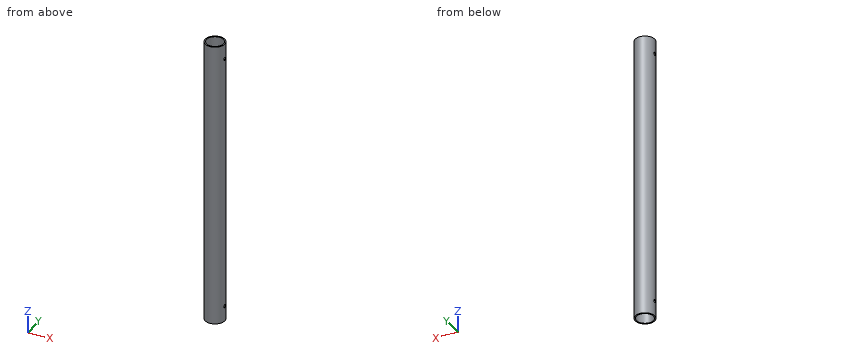
from build123d import *

# Parameters (mm, degrees)
F0_R          = 15.875
F0_R_2        = 13.875
F1_DEPTH      = 470
F2_R          = 2.5
F3_DEPTH      = 30
F3_DEPTH_BACK = 30
F4_R          = 2.5
F5_DEPTH      = 25
F5_DEPTH_BACK = 25


with BuildPart() as f1:
    # F0 (on Top) → F1 (new body)
    with BuildSketch(Plane.XY):
        Circle(F0_R)
        Circle(F0_R_2, mode=Mode.SUBTRACT)
    extrude(amount=F1_DEPTH)

    # F2 (on Right) → F3 (cut, two sides)
    with BuildSketch(Plane.YZ) as f3_sk:
        with Locations((0, 25)):
            Circle(F2_R)
    extrude(amount=F3_DEPTH, mode=Mode.SUBTRACT)
    extrude(f3_sk.sketch, amount=-F3_DEPTH_BACK, mode=Mode.SUBTRACT)

    # F4 (on Right) → F5 (cut, two sides)
    with BuildSketch(Plane.YZ) as f5_sk:
        with Locations((0, 445)):
            Circle(F4_R)
    extrude(amount=-F5_DEPTH, mode=Mode.SUBTRACT)
    extrude(f5_sk.sketch, amount=F5_DEPTH_BACK, mode=Mode.SUBTRACT)


solid = f1.part
Input: part model. Units: mm. Frame: model coordinates. Give positions to 0.01 mm unless a question says otherwise; leave off trailing zeros. Order: outer loops, then holes, each group sorted by start corner. A loop starts at its lowest first (then second) coordinate and runs counter-clockwise, first axis right, second up. Notation, with made-up numbers: M 38.5,7 L 53.5,7 A16 cw 53.5,15 Z; hole C -27.5,64 d7. An arc over 180 degrees is marked long. Answer as a JSON object with one key per item and string values.
1. Ray query, line 1 (Z direction, x = 15.3, y = 0); line 2 (X direction, y = -1.5, z = 406); line 3 (Y direction, x = 0, z = 104.5) (3 decimals). Return the intervals inside material, ascending. Write a range as [from, to].
Result sheet:
{"line 1": "[0, 22.5], [27.5, 442.5], [447.5, 470]", "line 2": "[-15.8, -13.79], [13.79, 15.8]", "line 3": "[-15.875, -13.875], [13.875, 15.875]"}
2. Cut plane A-A, the plane x = 0. Output: boundary loops of the cut face in (y, z) (3 decimals), and give its area (3 significant figures).
Result sheet:
{"outline": "M -15.875,0 L -13.875,0 L -13.875,470 L -15.875,470 Z; M 13.875,0 L 15.875,0 L 15.875,470 L 13.875,470 Z", "area": "1,880 mm²"}
3. Cut plane B-B, the plane y = 9. Output: boundary loops of the cut face in (x, z).
Result sheet:
{"outline": "M -13.08,0 L -10.56,0 L -10.56,470 L -13.08,470 Z; M 10.56,0 L 13.08,0 L 13.08,470 L 10.56,470 Z"}
4. First-contact query: P1, Ø3, axis at y = 0, z = 25, coming from the +X side; P2, Ø3, axis at x = -8.5, z = 188, coming from the -Y side; P3, Ø4, axis at y = 5, z = 361.5, coming from the +X side; P4, Ø6, axis at y = -11.5, z = 310, coming from the -X side. Flat tips, straight axial feed; report the tip coordinate or a pass-through.
Result sheet:
{"P1": "through", "P2": "y = -14.25", "P3": "x = 15.59", "P4": "x = -13.41"}
5. Cut plane C-C, the plane z = 388. Output: boundary loops of the cut face in (x, y) (3 decimals), and give its area (3 significant figures).
Result sheet:
{"outline": "C 0,0 d31.75; hole C 0,0 d27.75", "area": "187 mm²"}
